Job drawing, mm, ordinate dimensions from the low corner. One solid piece. Round coordinates to 2 decimals unless told otherwise and drop trailing zeros. Loops run counter-clockwise (first coordinate to the right, second up) from the corner with the lowest first, then second, coordinate; pieces in that order, holes last.
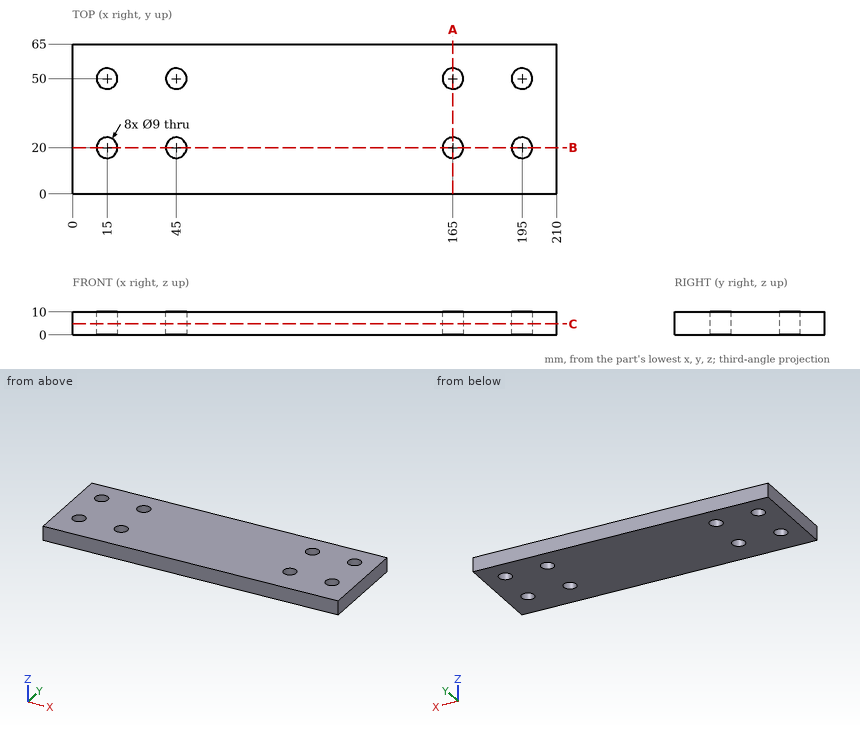
(1) Probe line 1 (Y direction, x = 15, z = 3.5); line 2 (X direction, y = 23, z = 8.5); line 3 (Y direction, x = 13.5, z = 3). List the from-to ranges inside material, lowest first.
Responses:
line 1: y = 0 to 15.5, 24.5 to 45.5, 54.5 to 65
line 2: x = 0 to 11.65, 18.35 to 41.65, 48.35 to 161.65, 168.35 to 191.65, 198.35 to 210
line 3: y = 0 to 15.76, 24.24 to 45.76, 54.24 to 65
(2) Slice it at C-C on z = 4.75. Count the separate pieces of the cut face and the enclosed holes in it, plus the area to 3 significant figures.
Responses:
separate pieces: 1
enclosed holes: 8
area: 13,100 mm2
(3) Slice it at A-A on x = 165. List the corners of the cut face in (y, z), plus the area to 3 significant figures.
Responses:
outline: (0, 0) - (15.5, 0) - (15.5, 10) - (0, 10) - close; (24.5, 0) - (45.5, 0) - (45.5, 10) - (24.5, 10) - close; (54.5, 0) - (65, 0) - (65, 10) - (54.5, 10) - close
area: 470 mm2
(4) Slice it at B-B on y = 20. List the corners of the cut face in (x, z).
Responses:
outline: (0, 0) - (10.5, 0) - (10.5, 10) - (0, 10) - close; (19.5, 0) - (40.5, 0) - (40.5, 10) - (19.5, 10) - close; (49.5, 0) - (160.5, 0) - (160.5, 10) - (49.5, 10) - close; (169.5, 0) - (190.5, 0) - (190.5, 10) - (169.5, 10) - close; (199.5, 0) - (210, 0) - (210, 10) - (199.5, 10) - close
